Design review of the part built by this model. Coordinates are the model's own, in mm. Give positions to 0.01 mm unless a question says otherwise; leave off trailing zeros. Order: outer loops, then holes, each group sorted by start corner. A loop starts at its lowest first (then second) coordinate and runs counter-clockwise, first axis right, second up. Notation, with made-up numbers: M 39,89.5 L 78,89.5 A21 ccw 78,126.5 Z; hole C -31,77 d2. An arc over 180 degrees is marked long. Answer as a JSON object with one key per item and string values.
from build123d import *

# Parameters (mm, degrees)
SKETCH1_R           = 2.3495
SKETCH1_R_2         = 4.445
BOSS_EXTRUDE1_DEPTH = 2.54
SKETCH2_R           = 2.413
CUT_EXTRUDE1_DEPTH  = 217.884748371
SKETCH3_W           = 16.89488816
SKETCH3_H           = 31.623
CUT_EXTRUDE2_DEPTH  = 217.884748371
SKETCH4_W           = 12.77569874
SKETCH4_H           = 24.435209008
SKETCH4_W_2         = 40.233428475
SKETCH4_H_2         = 28.333759116
CUT_EXTRUDE3_DEPTH  = 217.884748371
SKETCH5_R           = 2.413
CUT_EXTRUDE4_DEPTH  = 217.884748371


with BuildPart() as part:
    # Sketch1 → Boss-Extrude1 (new body)
    with BuildSketch(Plane.XY):
        Polygon((-2.930050059, -104.509781075), (-3.314938219, -104.509781075), (-3.314938219, -110.859781075), (-3.314938219, -123.559781075), (-2.930050059, -123.559781075), (-2.930050059, -168.708281075), (38.709428475, -168.708281075), (38.709428475, -189.536281075), (105.397061781, -189.536281075), (66.517436481, -110.859781075), (45.329949941, -110.859781075), (45.329949941, -104.509781075), (45.329949941, -72.886781075), (45.329949941, -66.536781075), (66.517436481, -66.536781075), (105.397061781, 12.139718925), (38.709428475, 12.139718925), (38.709428475, -8.688281075), (-2.930050059, -8.688281075), (-2.930050059, -53.836781075), (-3.314938219, -53.836781075), (-3.314938219, -66.536781075), (-3.314938219, -72.886781075), (-2.930050059, -72.886781075), align=None)
        with Locations((90.673911143, 2.614718925)):
            Circle(SKETCH1_R, mode=Mode.SUBTRACT)
        with Locations((41.95655448, -16.435281075)):
            Circle(SKETCH1_R, mode=Mode.SUBTRACT)
        with Locations((3.035061781, -60.186781075)):
            Circle(SKETCH1_R, mode=Mode.SUBTRACT)
        with Locations((3.035061781, -117.209781075)):
            Circle(SKETCH1_R, mode=Mode.SUBTRACT)
        with Locations((41.95655448, -160.961281075)):
            Circle(SKETCH1_R, mode=Mode.SUBTRACT)
        with Locations((90.673911143, -180.011281075)):
            Circle(SKETCH1_R, mode=Mode.SUBTRACT)
        with Locations((51.409428475, -3.100281075)):
            Circle(SKETCH1_R_2, mode=Mode.SUBTRACT)
    extrude(amount=BOSS_EXTRUDE1_DEPTH)

    # Sketch2 → Cut-Extrude1 (cut, through all)
    with BuildSketch(Plane.XY.offset(2.54)):
        with Locations((9.385061781, -69.711781075)):
            Circle(SKETCH2_R)
        with Locations((34.785061781, -69.711781075)):
            Circle(SKETCH2_R)
        with Locations(Location((34.785061781, -107.684781075, 0), (0, 0, 180))):
            Circle(SKETCH2_R)
        with Locations(Location((9.385061781, -107.684781075, 0), (0, 0, 180))):
            Circle(SKETCH2_R)
    extrude(amount=-CUT_EXTRUDE1_DEPTH, mode=Mode.SUBTRACT)

    # Sketch3 → Cut-Extrude2 (cut, through all)
    with BuildSketch(Plane.XY.offset(2.54)):
        with Locations((36.882505861, -88.698281075)):
            Rectangle(SKETCH3_W, SKETCH3_H)
    extrude(amount=-CUT_EXTRUDE2_DEPTH, mode=Mode.SUBTRACT)

    # Sketch4 → Cut-Extrude3 (cut, through all)
    with BuildSketch(Plane.XY.offset(2.54)):
        with Locations((33.845579105, 3.529323429)):
            Rectangle(SKETCH4_W, SKETCH4_H)
        with Locations((20.116714238, -182.875160633)):
            Rectangle(SKETCH4_W_2, SKETCH4_H_2)
    extrude(amount=-CUT_EXTRUDE3_DEPTH, mode=Mode.SUBTRACT)

    # Sketch5 → Cut-Extrude4 (cut, through all)
    with BuildSketch(Plane(origin=(0, 0, 0), x_dir=(-1, 0, 0), z_dir=(0, 0, -1))):
        with Locations((-32.121949941, -22.404281075)):
            Circle(SKETCH5_R)
        with Locations((-32.121949941, -56.694281075)):
            Circle(SKETCH5_R)
    extrude(amount=-CUT_EXTRUDE4_DEPTH, mode=Mode.SUBTRACT)


solid = part.part
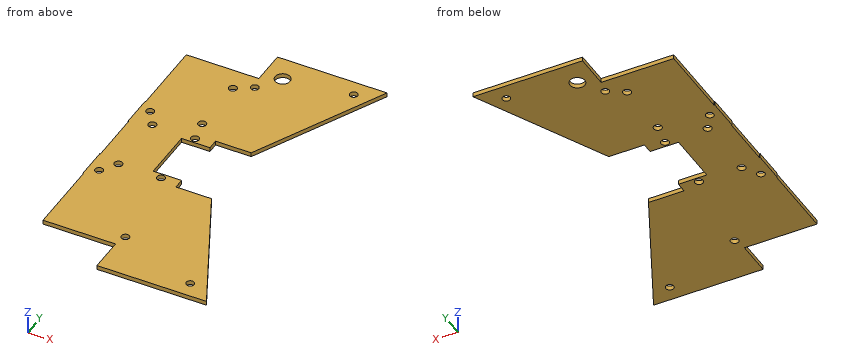
(1) We need section A-A (x = 69). Write out the cut boundary in (y, z).
Checked values:
{"outline": "M -189.54,0 L -115.88,0 L -115.88,2.54 L -189.54,2.54 Z; M -61.51,0 L 12.14,0 L 12.14,2.54 L -61.51,2.54 Z"}
(2) We need section D-D (y = -135). Write out the cut boundary in (x, z).
Checked values:
{"outline": "M -2.93,0 L 78.45,0 L 78.45,2.54 L -2.93,2.54 Z"}
(3) We need section C-C (z = 1.3). Count the separate pieces of the cut face and the enclosed holes in it, plus the area to 3 significant figures.
Checked values:
{"separate pieces": "1", "enclosed holes": "13", "area": "13,500 mm^2"}
(4) Insertion check: pin 1 (1.5 mm diameter, centred on y = -142.5, z = 2, fed in from -X); pin 2 (1.3 mm diameter, centred on x = 11, z = 1.5, fed in from +Y); pin 3 (4 mm diameter, centred on x = 90.67, y = -180.01, fed in from +Z). Each pin has a flat end and moves straight along its axis. Give the tip position at first contact, or say it passes through.
Checked values:
{"pin 1": "stops at x = -2.93", "pin 2": "stops at y = -8.69", "pin 3": "passes through"}
(5) We need section B-B (x = 15). Write out the cut boundary in (y, z), plus the area to 3 significant figures.
Checked values:
{"outline": "M -168.71,0 L -8.69,0 L -8.69,2.54 L -168.71,2.54 Z", "area": "406 mm^2"}
(6) To check wall thickness, follow L1, parallel to Y at x = 32, z = 1.15; L2, parallel to Y at x = 39, z = 0.6; L3, parallel to Y at x = 48, z = 1.05. State the ranges of each line that lie inside material, in increasing order. Write a range as from..to.
Checked values:
{"L1": "y = -168.71..-104.51, -72.89..-59.1, -54.28..-24.81, -19.99..-8.69", "L2": "y = -168.71..-104.51, -72.89..-8.69", "L3": "y = -189.54..-110.86, -66.54..-5.95, -0.25..12.14"}
